Geometry check sheet. Reference: the model listing, model coordinates, mm. A direction names the side the tool comes from. Give positions to 0.01 mm unless a question says otherwise; leave off trailing zeros. Order: outer loops, then holes, each group sorted by start corner. A loop starts at its lowest first (then second) coordinate and runs counter-clockwise, first axis right, second up.
```python
from build123d import *

# Parameters (mm, degrees)
SKETCH_1_W                       = 25
SKETCH_1_H                       = 32
SM_BASE_FLANGE_1_DEPTH           = 3
SM_EDGE_FLANGE_1_STRIP_W         = 13.4732
SM_EDGE_FLANGE_1_STRIP_H         = 3
SM_EDGE_FLANGE_1_STRIP_CUT_DEPTH = 25
SM_EDGE_FLANGE_1_DEPTH           = 25
SKETCH_13_R                      = 10.25
CUT_EXTRUDE_1_DEPTH              = 10
SKETCH_15_R                      = 1.5
CUT_EXTRUDE_2_DEPTH              = 10
FILLET_1_R                       = 10
FILLET_2_R                       = 5


# Sheet-metal steps are written as plain solids
with BuildPart() as part:
    # Sketch 1 → 基体-法兰1 (new body)
    with BuildSketch(Plane.XY):
        Rectangle(SKETCH_1_W, SKETCH_1_H)
    extrude(amount=-SM_BASE_FLANGE_1_DEPTH)

    # 边线-法兰1 strip (across the edge) → 边线-法兰1 strip cut (cut)
    with BuildSketch(Plane(origin=(-12.5, -16, 0), x_dir=(0, 1, 0), z_dir=(1, 0, 0))):
        with Locations((-3, -1.5)):
            Rectangle(SM_EDGE_FLANGE_1_STRIP_W, SM_EDGE_FLANGE_1_STRIP_H)
    extrude(amount=SM_EDGE_FLANGE_1_STRIP_CUT_DEPTH, mode=Mode.SUBTRACT)

    # 边线-法兰1 section (across the edge) → 边线-法兰1 (add)
    with BuildSketch(Plane(origin=(-12.5, -16, 0), x_dir=(0, 1, 0), z_dir=(1, 0, 0))):
        with BuildLine():
            Line((0, 0.7366), (0, 12))
            Line((0, 12), (3, 12))
            Line((3, 12), (3, 0.7366))
            ThreePointArc((3, 0.7366), (3.215745145, 0.215745145), (3.7366, 0))
            Line((3.7366, 0), (3.7366, -3))
            ThreePointArc((3.7366, -3), (1.094424801, -1.905575199), (0, 0.7366))
        make_face()
    extrude(amount=SM_EDGE_FLANGE_1_DEPTH)

    # 草图13 → 切除-拉伸1 (cut)
    with BuildSketch(Plane.XY):
        with Locations((0, 1)):
            Circle(SKETCH_13_R)
    extrude(amount=-CUT_EXTRUDE_1_DEPTH, mode=Mode.SUBTRACT)

    # 草图15 → 切除-拉伸2 (cut)
    with BuildSketch(Plane(origin=(0, -13, 0), x_dir=(1, 0, 0), z_dir=(0, 1, 0))):
        with Locations(Location((-7.5, -6, 0), (0, 0, 270))):
            Circle(SKETCH_15_R)
        with Locations(Location((7.5, -6, 0), (0, 0, 270))):
            Circle(SKETCH_15_R)
    extrude(amount=-CUT_EXTRUDE_2_DEPTH, mode=Mode.SUBTRACT)

    # 圆角1
    fillet_1_edges = [part.edges().sort_by_distance(p)[0] for p in [
        (-12.5, 16, -1.5),
        (12.5, 16, -1.5),
    ]]
    fillet(fillet_1_edges, radius=FILLET_1_R)

    # 圆角2
    fillet_2_edges = [part.edges().sort_by_distance(p)[0] for p in [
        (-12.5, -14.5, 12),
        (12.5, -14.5, 12),
    ]]
    fillet(fillet_2_edges, radius=FILLET_2_R)


solid = part.part
```
Q1. Cross-section at D-D, the plane x = 7. Record the boundary of the cut face in (y, z), and give its area (3 significant figures).
Q2. Cross-section at A-A, the plane x = 0. Record the boundary of the cut face in (y, z).
Q3. Access from +Z, -Z, +X, -X, +Y, -Y to the whole of each face (thin tool, end or side, straight path). Record for faces 1 (the face through (0, -13, 6)), 2 (the face through (11, -14.48, 10.57)).
Q4. Thickness scan on L1, parallel to X at y = -14.8, z = 6; L2, parallel to Y at x = 4.25, z = 10.75; L3, parallel to Z at x = -3.75, y = 13. Record the ranges inside material, lowest first.
Q5. Cross-section at B-B, the plane y = 1. Record the boundary of the cut face in (x, z), and give its area (3 significant figures).
Q6. Cross-section at C-C, the plane z = 6. Record the boundary of the cut face in (x, y), and give its area (3 significant figures).
Q7. Gauge pin test, flat ends, axial feed: P1, Ø3.5, axis at x = 1.5, z = 8.5, coming from the +Y side; P2, Ø4, axis at y = -10.5, z = 2.5, coming from the +X side; P3, Ø7.5, axis at x = -2.5, y = 8.5, coming from the +Z side. Record the tip position at first contact, or that the pin passes through.
Q8. Release check for a two-part mould opening along X. For faces 3 (the face through (9.65, 12.99, -1.52)), 4 (the face through (-9, -14, 6)), 5 (the face through (-0.2, 11.5, -3)) record: pulls with the +X half, pulls with the -X half, needs draft (parallel to the pull), parting line crosses it, or undercut.
Answers follow:
1. outline: (-16, 0.74) arc R3.74 ccw to (-12.26, -3) - (-6.49, -3) - (-6.49, 0) - (-12.26, 0) arc R0.74 cw to (-13, 0.74) - (-13, 4.59) - (-16, 4.59) - close; (-16, 7.41) - (-13, 7.41) - (-13, 12) - (-16, 12) - close; (8.49, -3) - (14.93, -3) - (14.93, 0) - (8.49, 0) - close
1. area: 72.5 mm2
2. outline: (-16, 0.74) arc R3.74 ccw to (-12.26, -3) - (-9.25, -3) - (-9.25, 0) - (-12.26, 0) arc R0.74 cw to (-13, 0.74) - (-13, 12) - (-16, 12) - close; (11.25, -3) - (16, -3) - (16, 0) - (11.25, 0) - close
3. face 1: +Z, +X, -X, +Y
3. face 2: +Z, +X, +Y, -Y
4. L1: x = -12.5 to -9, -6 to 6, 9 to 12.5
4. L2: y = -16 to -13
4. L3: z = -3 to 0
5. outline: (-12.5, -3) - (-10.25, -3) - (-10.25, 0) - (-12.5, 0) - close; (10.25, -3) - (12.5, -3) - (12.5, 0) - (10.25, 0) - close
5. area: 13.5 mm2
6. outline: (-12.5, -16) - (-9, -16) - (-9, -13) - (-12.5, -13) - close; (-6, -16) - (6, -16) - (6, -13) - (-6, -13) - close; (9, -16) - (12.5, -16) - (12.5, -13) - (9, -13) - close
6. area: 57.0 mm2
7. P1: stops at y = -13
7. P2: passes through
7. P3: stops at z = 0
8. face 3: pulls with the +X half
8. face 4: undercut
8. face 5: needs draft
